Here's how the part is built. I have some questions about the finished solid (model axes, mm). A direction names the side the tool comes from. Coordinates: 2 decimals unless noted, no trailing zeros. Write each loop counter-clockwise with the first axis right and the second up, starting at its lowest first coordinate (ties: lowest second). Pieces come first, ordered by that corner, then holes. Notation, with made-up numbers: (7.5, 60) - (28.5, 60) arc R14 ccw to (28.5, 71) - close; hole circle Ø4 at (-6, 61.25). An arc over 180 degrees is marked (long way). Answer in a Markdown table with one row per item. Add a question column.
Item 1: Imagine slicing it at D-D (y = 27). Please give me the cut outline in (x, z), plus the area to 3 significant figures.
Item 2: Imagine slicing it at A-A (x = 40). Please give me the cut outline in (y, z).
Item 3: If I drill on probe 1 along Z at (x, y) = (40, 5); probe 2 along Y at (x, z) = (11.5, -7.5); probe 3 along X at (y, z) = (22.5, -31), over which ranges is the centre line in solid material (lowest first)? Write a range as from..to.
Item 4: I'm going to push flat-ended pins straight in: pin 1 (7 mm diameter, centred on x = 40, z = -27, fed in from +Y); pin 2 (3 mm diameter, centred on y = 30, z = -26.5, fed in from +X); pin 3 (12.5 mm diameter, centred on x = 22, z = -11, fed in from +Y). Where does each tip first touch, or does it pass through?
Item 5: Which directions (+Z, -Z, +X, -X, +Y, -Y) give clear straight access to the entire face, cutting with the end or side of a thin tool? Please do faces 1 (the face through (40, 9, -17)), 2 (the face through (42.747, 4.563, -6.879)), 3 (the face through (17.18, 16.87, -16.76)).
Item 6: We'd pull the mould along Z, two halves only. Please class faces 4 (the face through (42.747, 4.563, -26.879)), 5 (the face through (9, 39, -17)), 6 (the face through (14, 9, -34)): +Z half, -Z half, draft (parallel to the pull), parting line (faces both ways), or undercut.
from build123d import *

# Parameters (mm, degrees)
EXTRUDE_11_DEPTH     = 34
SKETCH_32_R          = 2.75
CUT_EXTRUDE_21_DEPTH = 74.054773971
SKETCH_33_R          = 2.75
CUT_EXTRUDE_22_DEPTH = 74.054773971


with BuildPart() as part:
    # Sketch 31 → Extrude 11 (new body)
    with BuildSketch(Plane.XY):
        with BuildLine():
            Line((9, 30), (9, 49))
            ThreePointArc((9, 49), (8.707106781, 49.707106781), (8, 50))
            Line((8, 50), (1, 50))
            ThreePointArc((1, 50), (0.292893219, 49.707106781), (0, 49))
            Line((0, 49), (0, 1))
            ThreePointArc((0, 1), (0.292893219, 0.292893219), (1, 0))
            Line((1, 0), (49, 0))
            ThreePointArc((49, 0), (49.707106781, 0.292893219), (50, 1))
            Line((50, 1), (50, 8))
            ThreePointArc((50, 8), (49.707106781, 8.707106781), (49, 9))
            Line((49, 9), (30, 9))
            Line((30, 9), (9, 30))
        make_face()
        with BuildLine():
            Line((5.5, 12), (7.428034206, 12))
            ThreePointArc((7.428034206, 12), (7.761575809, 12.12750839), (7.925, 12.445000002))
            ThreePointArc((7.925, 12.445000002), (9.455281372, 15.213766146), (12.501000023, 16.068999997))
            ThreePointArc((12.501000023, 16.068999997), (12.854580588, 15.852403205), (12.923122843, 15.443459021))
            Line((12.923122843, 15.443459021), (12.661152875, 14.464571239))
            ThreePointArc((12.661152875, 14.464571239), (12.468861163, 14.187031274), (12.143999993, 14.095))
            ThreePointArc((12.143999993, 14.095), (10.514573143, 10.515407625), (14.095, 12.143000006))
            ThreePointArc((14.095, 12.143000006), (14.186987516, 12.467511304), (14.464129015, 12.659766017))
            Line((14.464129015, 12.659766017), (15.443998772, 12.92299967))
            ThreePointArc((15.443998772, 12.92299967), (15.853205766, 12.854713962), (16.069999999, 12.501000008))
            ThreePointArc((16.069999999, 12.501000008), (15.215158243, 9.454636454), (12.446, 7.924))
            ThreePointArc((12.446, 7.924), (12.127844119, 7.76084071), (12, 7.426924553))
            Line((12, 7.426924553), (12, 5.5))
            ThreePointArc((12, 5.5), (12.146446609, 5.146446609), (12.5, 5))
            Line((12.5, 5), (27.842893456, 5))
            ThreePointArc((27.842893456, 5), (28.30483088, 5.308653143), (28.196454654, 5.853545371))
            Line((28.196454654, 5.853545371), (5.853561034, 28.197438986))
            ThreePointArc((5.853561034, 28.197438986), (5.308663433, 28.305835138), (5, 27.843893575))
            Line((5, 27.843893575), (5, 12.5))
            ThreePointArc((5, 12.5), (5.146446609, 12.146446609), (5.5, 12))
        make_face(mode=Mode.SUBTRACT)
    extrude(amount=-EXTRUDE_11_DEPTH)

    # Sketch 32 → Cut-Extrude 21 (cut, through all)
    with BuildSketch(Plane(origin=(0, 9, 0), x_dir=(1, 0, 0), z_dir=(0, 1, 0))):
        with Locations(Location((40, 27, 0), (0, 0, 180))):
            Circle(SKETCH_32_R)
        with Locations(Location((40, 7, 0), (0, 0, 180))):
            Circle(SKETCH_32_R)
    extrude(amount=-CUT_EXTRUDE_21_DEPTH, mode=Mode.SUBTRACT)

    # Sketch 33 → Cut-Extrude 22 (cut, through all)
    with BuildSketch(Plane(origin=(9, 0, 0), x_dir=(0, 0, -1), z_dir=(1, 0, 0))):
        with Locations(Location((7, 40, 0), (0, 0, 90))):
            Circle(SKETCH_33_R)
        with Locations(Location((27, 40, 0), (0, 0, 90))):
            Circle(SKETCH_33_R)
    extrude(amount=-CUT_EXTRUDE_22_DEPTH, mode=Mode.SUBTRACT)


solid = part.part
Here are the results:
| question | item | result |
|---|---|---|
| 1 | outline | (0, -34) - (5, -34) - (5, 0) - (0, 0) - close; (7.05, -34) - (12, -34) - (12, 0) - (7.05, 0) - close |
| 1 | area | 338 mm2 |
| 2 | outline | (0, -34) - (9, -34) - (9, -29.75) - (0, -29.75) - close; (0, -24.25) - (9, -24.25) - (9, -9.75) - (0, -9.75) - close; (0, -4.25) - (9, -4.25) - (9, 0) - (0, 0) - close |
| 3 | probe 1 | z = -34..-29.75, -24.25..-9.75, -4.25..0 |
| 3 | probe 2 | y = 0..9.96, 14.04..16.07, 22.55..27.5 |
| 3 | probe 3 | x = 0..5, 11.55..16.5 |
| 4 | pin 1 | stops at y = 9 |
| 4 | pin 2 | stops at x = 10.5 |
| 4 | pin 3 | stops at y = 23.25 |
| 5 | face 1 | +Z, -Z, +X, +Y |
| 5 | face 2 | +Y, -Y |
| 5 | face 3 | +Z, -Z |
| 6 | face 4 | undercut |
| 6 | face 5 | draft |
| 6 | face 6 | -Z half |
